from build123d import *

# Parameters (mm, degrees)
F0_R     = 6
F0_R_2   = 1.65
F1_DEPTH = 3
F2_R     = 6
F3_DEPTH = 5.5
F5_DEPTH = 3
F6_R     = 0.5
F7_R     = 2.75
F8_DEPTH = 5


with BuildPart() as f1:
    # F0 (on Top) → F1 (new body)
    with BuildSketch(Plane.XY):
        Circle(F0_R)
        with Locations((-3.175, 0)):
            Circle(F0_R_2, mode=Mode.SUBTRACT)
        with Locations((3.175, 0)):
            Circle(F0_R_2, mode=Mode.SUBTRACT)
    extrude(amount=F1_DEPTH)

    # F2 (on face) → F3 (join)
    with BuildSketch(Plane(origin=(0, 0, 0), x_dir=(1, 0, 0), z_dir=(0, 0, -1))):
        Circle(F2_R)
    extrude(amount=F3_DEPTH)

    # F4 (on face) → F5 (cut)
    with BuildSketch(Plane.XY.offset(3)):
        with BuildLine():
            ThreePointArc((3.968627, 4.5), (0, 6), (-3.968627, 4.5))
            Line((-3.968627, 4.5), (-1.968627, 4.5))
            Line((-1.968627, 4.5), (-1.968627, 2.5))
            Line((-1.968627, 2.5), (1.968627, 2.5))
            Line((1.968627, 2.5), (1.968627, 4.5))
            Line((1.968627, 4.5), (3.968627, 4.5))
        make_face()
    extrude(amount=-F5_DEPTH, mode=Mode.SUBTRACT)

    # F6
    f6_edges = [f1.edges().sort_by_distance(p)[0] for p in [
        (-3.968627, 4.5, 1.5),
        (-1.968627, 4.5, 1.5),
        (1.968627, 2.5, 1.5),
        (1.968627, 4.5, 1.5),
        (3.968627, 4.5, 1.5),
        (-1.968627, 2.5, 1.5),
    ]]
    fillet(f6_edges, radius=F6_R)

    # F7 (on face) → F8 (cut)
    with BuildSketch(Plane(origin=(0, 0, -5.5), x_dir=(1, 0, 0), z_dir=(0, 0, -1))):
        Circle(F7_R)
    extrude(amount=-F8_DEPTH, mode=Mode.SUBTRACT)


solid = f1.part
CAD build for the part. Positions are in the model's coordinates, mm. A direction names the side the tool comes from. Coordinates: 2 decimals unless noted, no trailing zeros. Write each loop counter-clockwise with the first axis right and the second up, starting at its lowest first coordinate (ties: lowest second). Pieces come first, ordered by that corner, then holes. Notation, with made-up numbers: M -34.5,60.25 L -2.5,60.25 A22 ccw -2.5,92.25 Z; hole C 41.5,73 d6. An arc over 180 degrees is marked long. Return JSON: item names as keys, results as strings.
Item 1: Slice it at D-D, the plane z = -3.5. Write the cut outline in (x, y), and give its area (3 significant figures).
Findings below:
{"outline": "C 0,0 d12; hole C 0,0 d5.5", "area": "89.3 mm2"}
Item 2: Slice it at B-B, the plane x = 0. Write the cut outline in (y, z).
Findings below:
{"outline": "M -6,-5.5 L -2.75,-5.5 L -2.75,-0.5 L 2.75,-0.5 L 2.75,-5.5 L 6,-5.5 L 6,0 L 2.5,0 L 2.5,3 L -6,3 Z"}
Item 3: Drop flat-ended pins along their axis: pin 1 Ø3 at (x, z) = (-4, 2) entering from +Y; pin 2 Ø0.9 at (x, z) = (0, 2) entering from +Y; pin 3 Ø1 at (x, y) = (3, -0.5) entering from +Z. Give the stop position or say it passes through.
Findings below:
{"pin 1": "stops at y = 4.5", "pin 2": "stops at y = 2.5", "pin 3": "stops at z = 0"}
Item 4: Slice it at C-C, the plane y = 0. Write the cut outline in (x, z) (3 decimals), and give its area (3 significant figures).
Findings below:
{"outline": "M -6,-5.5 L -2.75,-5.5 L -2.75,-0.5 L 2.75,-0.5 L 2.75,-5.5 L 6,-5.5 L 6,3 L 4.825,3 L 4.825,0 L 1.525,0 L 1.525,3 L -1.525,3 L -1.525,0 L -4.825,0 L -4.825,3 L -6,3 Z", "area": "54.7 mm2"}
Item 5: Slice it at A-A, the plane z = 0.75. Write the cut outline in (x, y) (3 decimals), and give its area (3 significant figures).
Findings below:
{"outline": "M -4.118,4.364 A6 ccw long 4.118,4.364 A0.5 ccw 3.775,4.5 L 2.469,4.5 A0.5 ccw 1.969,4 L 1.969,3 A0.5 cw 1.469,2.5 L -1.469,2.5 A0.5 cw -1.969,3 L -1.969,4 A0.5 ccw -2.469,4.5 L -3.775,4.5 A0.5 ccw Z; hole C -3.175,0 d3.3; hole C 3.175,0 d3.3", "area": "79.9 mm2"}
Item 6: Two-plate mould, pull along Y, no slides. Class faces 1 (the flat face through (-3, 4.5, 2)), 2 (the flat face through (0, 0, -0.5)), 3 (the flat face through (0, 4, 0)): +Y half, -Y half, draft (parallel to the pull), parting line (faces both ways), or undercut.
Findings below:
{"face 1": "+Y half", "face 2": "undercut", "face 3": "draft"}
Item 7: Probe line 1 (X direction, y = 0, z = -4); line 2 (Z direction, x = -1, y = -0.75). List the from-to ranges inside material, lowest first. Write a range as from..to.
Findings below:
{"line 1": "x = -6..-2.75, 2.75..6", "line 2": "z = -0.5..3"}
Item 8: Which spindle directions (+Z, -Z, +X, -X, +Y, -Y) get a long thin tool onto all of the face, cutting with end or side? Do faces 4 (the flat face through (3, 4.5, 2)), 5 (the cylindrical face through (1.527, 0.073, 1.479)), 6 (the flat face through (1.969, 3.5, 1.5)), 7 (the cylindrical face through (-0.596, 2.685, -3.035)). Say none if no direction does.
Findings below:
{"face 4": "+Z, +X, -X, +Y", "face 5": "+Z", "face 6": "+Z, +Y", "face 7": "-Z"}
